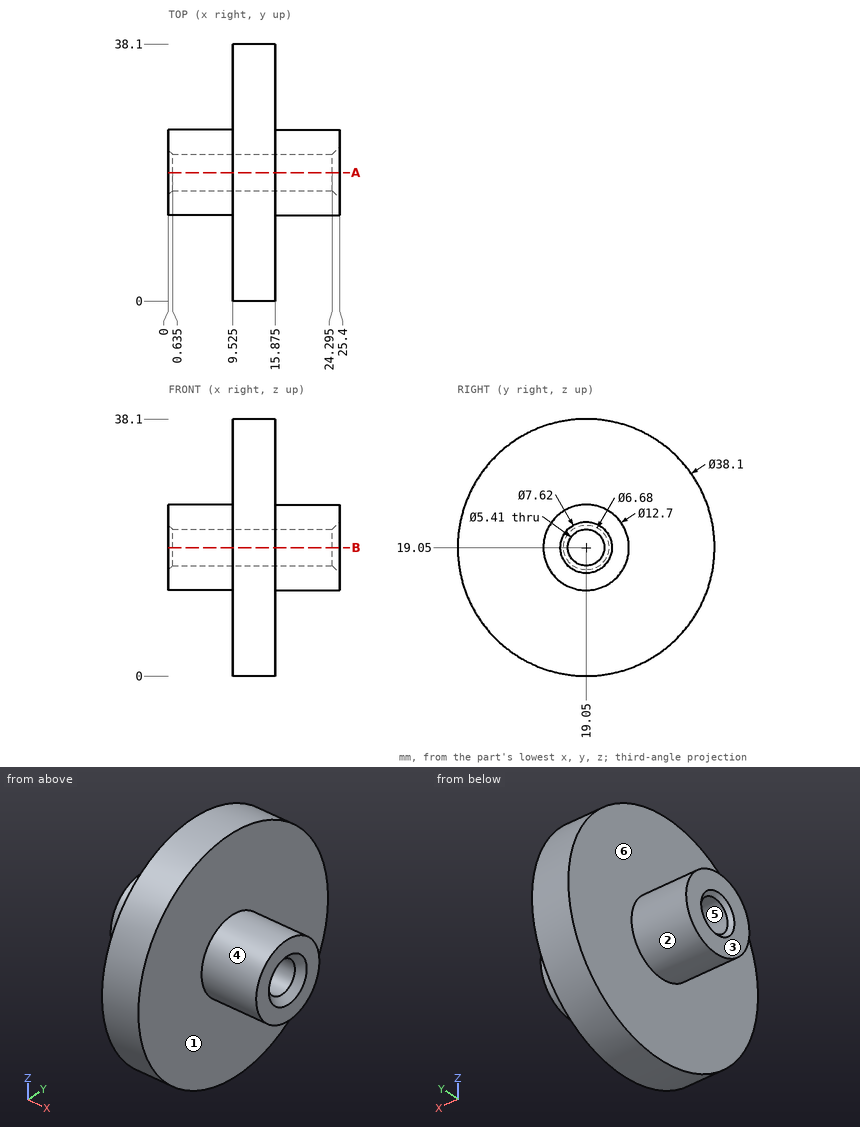
Study the drawing (mm; zero at the part's minimum x, y, z) and answer. A direction names the side the tool comes from. Coordinates: 2 decimals unless noted, no trailing zeros. Write each loop counter-clockwise with the first axis right and the second up, starting at its lowest first coordinate (ties: lowest second). Pieces come first, ordered by that corner, then holes. Notation, with made-up numbers: (83.25, 50) - (121.25, 50) arc R24 ccw to (121.25, 82) - close; hole circle Ø7 at (-3.5, -9). An arc over 180 degrees is marked (long way). Answer as a JSON object with one key per item and string values. Group by question number.
1. Which of the six approach directions +Z, -Z, +X, -X, +Y, -Y give full straight-line access (tool end or side, diameter ignored) to the marked faces 1, 2 and 3?
2. The mould has two halves that part along Z. Classify the marked faces 4, 5 and 6: +Z half, -Z half, draft (parallel to the pull), parting line (faces both ways), or undercut.
3. Consider L1, parallel to Y at x = 15.25, z = 19.05 (1 decimal); L2, parallel to Y at x = 1.5, z = 19 (1 decimal). Determine where each line is inside the solid, lowest interval first. Write a range as [from, to].
4. Each of these flat-tipped pins is pushed along its axis until it touches: P1, Ø5, axis at x = 8, y = 33, coming from the +Z side; P2, Ø10, axis at y = 7, z = 16, coming from the -X side (3 decimals); P3, Ø6, axis at x = 19, z = 6, coming from the +Y side; P4, Ø1, axis at x = 15, y = 32, coming from the -Z side. Where does it stop, or does it pass through?
5. A cutting plane is placed at A-A (y = 19.05). Determine the outline of the cut face in (x, z) (1 decimal).
Worked out:
{
 "1": {"face 1": "+X", "face 2": "-X", "face 3": "+Z, -Z, -X, +Y, -Y"},
 "2": {"face 4": "parting line", "face 5": "undercut", "face 6": "draft"},
 "3": {"L1": "y = [0, 16.3], [21.8, 38.1]", "L2": "y = [12.7, 16.3], [21.8, 25.4]"},
 "4": {"P1": "stops at z = 33.87", "P2": "stops at x = 9.525", "P3": "passes through", "P4": "stops at z = 4.63"},
 "5": {"outline": "(0, 12.7) - (9.5, 12.7) - (9.5, 0) - (15.9, 0) - (15.9, 12.7) - (25.4, 12.7) - (25.4, 15.2) - (24.3, 16.3) - (0.6, 16.3) - (0, 15.7) - close; (0, 22.4) - (0.6, 21.8) - (24.3, 21.8) - (25.4, 22.9) - (25.4, 25.4) - (15.9, 25.4) - (15.9, 38.1) - (9.5, 38.1) - (9.5, 25.4) - (0, 25.4) - close"}
}
